The listing builds one solid part. Answer for the finished solid, in the listing's coordinates (mm). Face numbers are marked on the shaded views. A direction names the side the tool comes from. Coordinates: 2 decimals unless noted, no trailing zeros. Loops run counter-clockwise (first coordinate to the right, second up) from the corner with the lowest first, then second, coordinate; pieces in that order, holes last. Notation, with made-up numbers: (70, -1.5) - (97, -1.5) arc R25 ccw to (97, 33.5) - close; hole circle Ø7 at (49, 12.25). An arc over 180 degrees is marked (long way). Put each result on its own line as item: value.
```python
from build123d import *

# Parameters (mm, degrees)
EXTRUDE_1_DEPTH          = 50
CUT_EXTRUDE_1_DEPTH      = 74.164198895
CUT_EXTRUDE_1_DEPTH_BACK = 74.164198895
SKETCH_2_R               = 2
SKETCH_3_R               = 3.5
CUT_EXTRUDE_2_DEPTH      = 2
CHAMFER_1_SIZE           = 1.5
CUT_EXTRUDE_3_DEPTH      = 3


with BuildPart() as part:
    # 스케치1 → 보스-돌출1 (new body)
    with BuildSketch(Plane.XY):
        with BuildLine():
            Line((-1.5, 32.465366161), (-1.5, 42))
            Line((-1.5, 42), (-8.5, 42))
            Line((-8.5, 42), (-8.5, 31.886517527))
            ThreePointArc((-8.5, 31.886517527), (0, -33), (8.5, 31.886517527))
            Line((8.5, 31.886517527), (8.5, 42))
            Line((8.5, 42), (1.5, 42))
            Line((1.5, 42), (1.5, 32.465366161))
            Line((1.5, 32.465366161), (1.5, 27.559208987))
            ThreePointArc((1.5, 27.559208987), (1.514407087, 27.558421057), (1.528813761, 27.557625596))
            ThreePointArc((1.528813761, 27.557625596), (8.110662779, 26.890433295), (14.48576204, 25.122951621))
            ThreePointArc((14.48576204, 25.122951621), (29, 0), (14.48576204, -25.122951621))
            ThreePointArc((14.48576204, -25.122951621), (8.110662779, -26.890433295), (1.528813761, -27.557625596))
            ThreePointArc((1.528813761, -27.557625596), (0, -27.6), (-1.528813761, -27.557625596))
            ThreePointArc((-1.528813761, -27.557625596), (-8.110662779, -26.890433295), (-14.48576204, -25.122951621))
            ThreePointArc((-14.48576204, -25.122951621), (-29, 0), (-14.48576204, 25.122951621))
            ThreePointArc((-14.48576204, 25.122951621), (-8.110662779, 26.890433295), (-1.528813761, 27.557625596))
            ThreePointArc((-1.528813761, 27.557625596), (-1.514407087, 27.558421057), (-1.5, 27.559208987))
            Line((-1.5, 27.559208987), (-1.5, 32.465366161))
        make_face()
    extrude(amount=EXTRUDE_1_DEPTH)

    # 스케치2 → 컷-돌출1 (cut, two sides: drawn at the far end of the back side and taken through both)
    with BuildSketch(Plane(origin=(0, 0, 0), x_dir=(0, 0, -1), z_dir=(1, 0, 0)).offset(-CUT_EXTRUDE_1_DEPTH_BACK)):
        with Locations(Location((-35, 36, 0), (0, 0, 90))):
            Circle(SKETCH_2_R)
        with Locations(Location((-15, 36, 0), (0, 0, 90))):
            Circle(SKETCH_2_R)
    extrude(amount=CUT_EXTRUDE_1_DEPTH + CUT_EXTRUDE_1_DEPTH_BACK, mode=Mode.SUBTRACT)

    # 스케치3 → 컷-돌출2 (cut)
    with BuildSketch(Plane.ZY.offset(8.5)):
        with Locations((15, 36)):
            Circle(SKETCH_3_R)
        with Locations((35, 36)):
            Circle(SKETCH_3_R)
    extrude(amount=-CUT_EXTRUDE_2_DEPTH, mode=Mode.SUBTRACT)

    # 모따기1
    chamfer_1_edges = [part.edges().sort_by_distance(p)[0] for p in [
        (-5, 42, 50),
        (5, 42, 0),
        (-5, 42, 0),
        (5, 42, 50),
        (8.5, 42, 25),
        (-8.5, 42, 25),
    ]]
    chamfer(chamfer_1_edges, length=CHAMFER_1_SIZE)

    # 스케치4 → 컷-돌출3 (cut)
    with BuildSketch(Plane(origin=(8.5, 0, 0), x_dir=(0, 0, -1), z_dir=(1, 0, 0))):
        Polygon((-30.785343035, 36), (-32.892671517, 39.65), (-37.107328483, 39.65), (-39.214656965, 36), (-37.107328483, 32.35), (-32.892671517, 32.35), align=None)
        Polygon((-10.785343035, 36), (-12.892671517, 39.65), (-17.107328483, 39.65), (-19.214656965, 36), (-17.107328483, 32.35), (-12.892671517, 32.35), align=None)
    extrude(amount=-CUT_EXTRUDE_3_DEPTH, mode=Mode.SUBTRACT)


solid = part.part
```
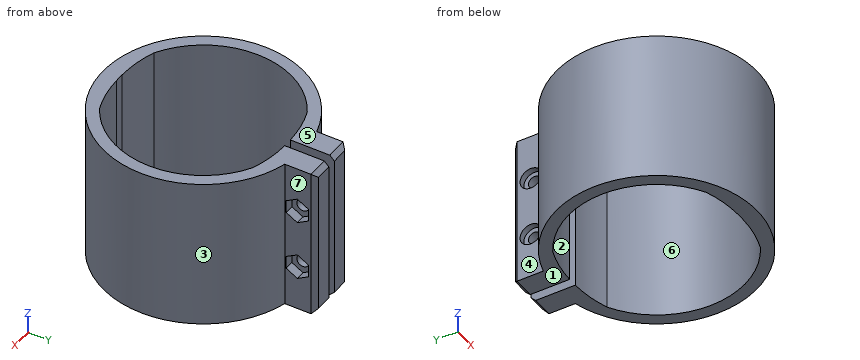
1) The part is cut by section A-A (z = 35). State how many separate pieces and enclosed holes the cut face has, and give its area (3 significant figures).
Found:
separate pieces: 3
enclosed holes: 0
area: 875 mm^2
2) The part is cut by section B-B (x = 9.5). Give the vertices of the cut face in (y, z), and give its area (3 significant figures).
Found:
outline: (-31.6, 0) - (-26.6, 0) - (-26.6, 50) - (-31.6, 50) - close; (26.6, 0) - (31.6, 0) - (31.6, 50) - (26.6, 50) - close
area: 500 mm^2
3) Straight lines are drawn through the part: L1, parallel to Z at x = -2.95, y = 36; L2, parallel to Y at x = -3.15, z = 15; L3, parallel to X at y = 34, z = 29. For each, find the intervals that lie inside material, in ascending order. Write a range as [from, to].
Found:
L1: z = [0, 13], [17, 33], [37, 50]
L2: y = [-32.85, -27.5], [27.5, 34], [38, 42]
L3: x = [-8.5, -1.5], [1.5, 8.5]
4) The part is cut by section C-C (y = 0). Give the vertices of the cut face in (x, z).
Found:
outline: (-33, 0) - (-29, 0) - (-29, 50) - (-33, 50) - close; (29, 0) - (33, 0) - (33, 50) - (29, 50) - close
5) Each of these flat-tipped pins is pushed along its axis until it touches: pin 1 (7.5 mm diameter, centred on y = 36.5, z = 14.5, fed in from -X); pin 2 (10 mm diameter, centred on x = -22.5, y = -21.5, fed in from -Z); pin 3 (3 mm diameter, centred on y = 36, z = 15, fed in from +X); pin 4 (0.9 mm diameter, centred on x = 6.5, z = 35, fed in from -Y). Where does it stop, or does it pass through?
Found:
pin 1: stops at x = -8.5
pin 2: stops at z = 0
pin 3: passes through
pin 4: stops at y = -32.44
6) For a pull along X with two mould halves and no side action, classify the marked faces 1, 2 and 3 as pulls with the +X half, pulls with the -X half, needs draft (parallel to the pull), parting line crosses it, or undercut.
Found:
face 1: needs draft
face 2: undercut
face 3: parting line crosses it
7) For the marked faces 4, 5, 6 and 7, determine the directions among +Z, -Z, +X, -X, +Y, -Y from which every point of the face is accessible in a straight line to the end or side of a thin tool.
Found:
face 4: +Z, -Z, -X, +Y
face 5: +Z, +X, -X, +Y, -Y
face 6: +Z, -Z
face 7: +Z, -Z, +X, +Y
